from build123d import *

# Parameters (mm, degrees)
SKETCH1_R           = 2.5
BOSS_EXTRUDE1_DEPTH = 5
SKETCH2_R           = 1.5
SKETCH2_W           = 50
SKETCH2_H           = 50
CUT_EXTRUDE1_DEPTH  = 5
SKETCH3_W           = 80
SKETCH3_H           = 300
CUT_EXTRUDE2_DEPTH  = 10
SKETCH5_R           = 3
CUT_EXTRUDE4_DEPTH  = 10
SKETCH4_R           = 3
CUT_EXTRUDE3_DEPTH  = 10


with BuildPart() as part:
    # Sketch1 → Boss-Extrude1 (new body)
    with BuildSketch(Plane.XY):
        with BuildLine():
            Line((-123.5, 121.5), (-123.5, -121.5))
            ThreePointArc((-123.5, -121.5), (-122.914213562, -122.914213562), (-121.5, -123.5))
            Line((-121.5, -123.5), (121.5, -123.5))
            ThreePointArc((121.5, -123.5), (122.914213562, -122.914213562), (123.5, -121.5))
            Line((123.5, -121.5), (123.5, 121.5))
            ThreePointArc((123.5, 121.5), (122.914213562, 122.914213562), (121.5, 123.5))
            Line((121.5, 123.5), (-121.5, 123.5))
            ThreePointArc((-121.5, 123.5), (-122.914213562, 122.914213562), (-123.5, 121.5))
        make_face()
        with Locations((-118.5, 118.5)):
            Circle(SKETCH1_R, mode=Mode.SUBTRACT)
        with Locations((118.5, 118.5)):
            Circle(SKETCH1_R, mode=Mode.SUBTRACT)
        with Locations((118.5, -118.5)):
            Circle(SKETCH1_R, mode=Mode.SUBTRACT)
        with Locations((-118.5, -118.5)):
            Circle(SKETCH1_R, mode=Mode.SUBTRACT)
    extrude(amount=BOSS_EXTRUDE1_DEPTH)

    # Sketch2 → Cut-Extrude1 (cut)
    with BuildSketch(Plane(origin=(0, 0, 0), x_dir=(-1, 0, 0), z_dir=(0, 0, -1))):
        with Locations((28.284271247, 28.284271247)):
            Circle(SKETCH2_R)
        with Locations((28.284271247, -28.284271247)):
            Circle(SKETCH2_R)
        with Locations((-28.284271247, -28.284271247)):
            Circle(SKETCH2_R)
        with Locations((-28.284271247, 28.284271247)):
            Circle(SKETCH2_R)
        Rectangle(SKETCH2_W, SKETCH2_H)
    extrude(amount=-CUT_EXTRUDE1_DEPTH, mode=Mode.SUBTRACT)

    # Sketch3 → Cut-Extrude2 (cut)
    with BuildSketch(Plane(origin=(0, 0, 0), x_dir=(-1, 0, 0), z_dir=(0, 0, -1))):
        with Locations((-120, 0)):
            Rectangle(SKETCH3_W, SKETCH3_H)
    extrude(amount=-CUT_EXTRUDE2_DEPTH, mode=Mode.SUBTRACT)

    # Sketch5 → Cut-Extrude4 (cut)
    with BuildSketch(Plane(origin=(0, 0, 0), x_dir=(-1, 0, 0), z_dir=(0, 0, -1))):
        with Locations((-67, 108.5)):
            Circle(SKETCH5_R)
        with Locations((-67, 78.5)):
            Circle(SKETCH5_R)
        with Locations((-67, -108.5)):
            Circle(SKETCH5_R)
        with Locations((-67, -78.5)):
            Circle(SKETCH5_R)
    extrude(amount=-CUT_EXTRUDE4_DEPTH, mode=Mode.SUBTRACT)

    # Sketch4 → Cut-Extrude3 (cut)
    with BuildSketch(Plane(origin=(0, 0, 0), x_dir=(-1, 0, 0), z_dir=(0, 0, -1))):
        with Locations((-93, 78.5)):
            Circle(SKETCH4_R)
        with Locations((-93, 108.5)):
            Circle(SKETCH4_R)
        with Locations((-93, -78.5)):
            Circle(SKETCH4_R)
        with Locations((-93, -108.5)):
            Circle(SKETCH4_R)
    extrude(amount=-CUT_EXTRUDE3_DEPTH, mode=Mode.SUBTRACT)


solid = part.part
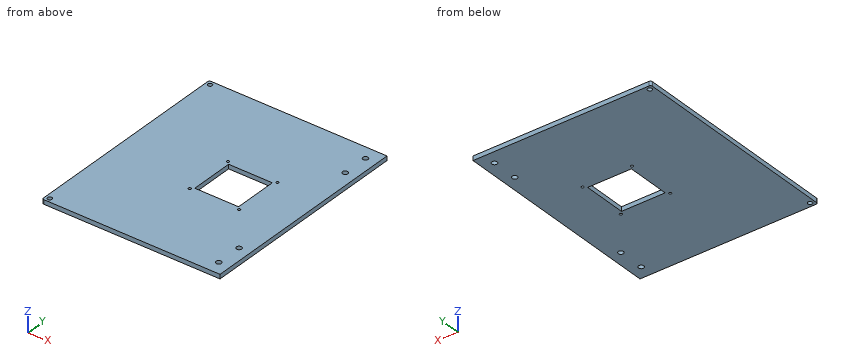
Source: CAD feature listing. Evaluate the final solid. Frame: model axes, mm. Coordinates: 2 decimals unless noted, no trailing zeros. Loops run counter-clockwise (first coordinate to the right, second up) from the corner with the lowest first, then second, coordinate; pieces in that order, holes last. Notation, with made-up numbers: (42, -9) - (91, -9) arc R22 cw to (91, -3) - close; hole circle Ø4 at (16.5, 73.25). An arc over 180 degrees is marked (long way). One line per item, written item: value. Start each with the question number.
1. Section A-A (x = -17). Return the cut outline in (y, z), and give its area (3 significant figures).
2. Ray query, L1, parallel to Y at x = -118.5, z = 1.1; L2, parallel to Y at x = 28, z = 3.25; L3, parallel to Y at x = 67, z = 2. Return the intervals inside material, ascending.
3. Contact query for flat-ended pins moving along their axis: P1, Ø3.5, axis at x = 67, y = -108.5, coming from the -Z side; P2, Ø10, axis at x = 5, y = 20.5, coming from the -Z side. Output: stop coordinate, or through.
4. Section C-C (z = 2.55). State how many separate pieces and enclosed holes the cut face has, and give its area (3 significant figures).
5. Section B-B (y = -108.5). Return the cut outline in (x, z), and give its area (4 significant figures).
Verdict:
1. outline: (-123.5, 0) - (-25, 0) - (-25, 5) - (-123.5, 5) - close; (25, 0) - (123.5, 0) - (123.5, 5) - (25, 5) - close
1. area: 985 mm2
2. L1: y = -123.5 to -121, -116 to 116, 121 to 123.5
2. L2: y = -123.5 to -29.76, -26.81 to 26.81, 29.76 to 123.5
2. L3: y = -123.5 to -111.5, -105.5 to -81.5, -75.5 to 75.5, 81.5 to 105.5, 111.5 to 123.5
3. P1: passes through
3. P2: stops at z = 0
4. separate pieces: 1
4. enclosed holes: 11
4. area: 47,600 mm2
5. outline: (-123.5, 0) - (64, 0) - (64, 5) - (-123.5, 5) - close; (70, 0) - (80, 0) - (80, 5) - (70, 5) - close
5. area: 987.5 mm2
